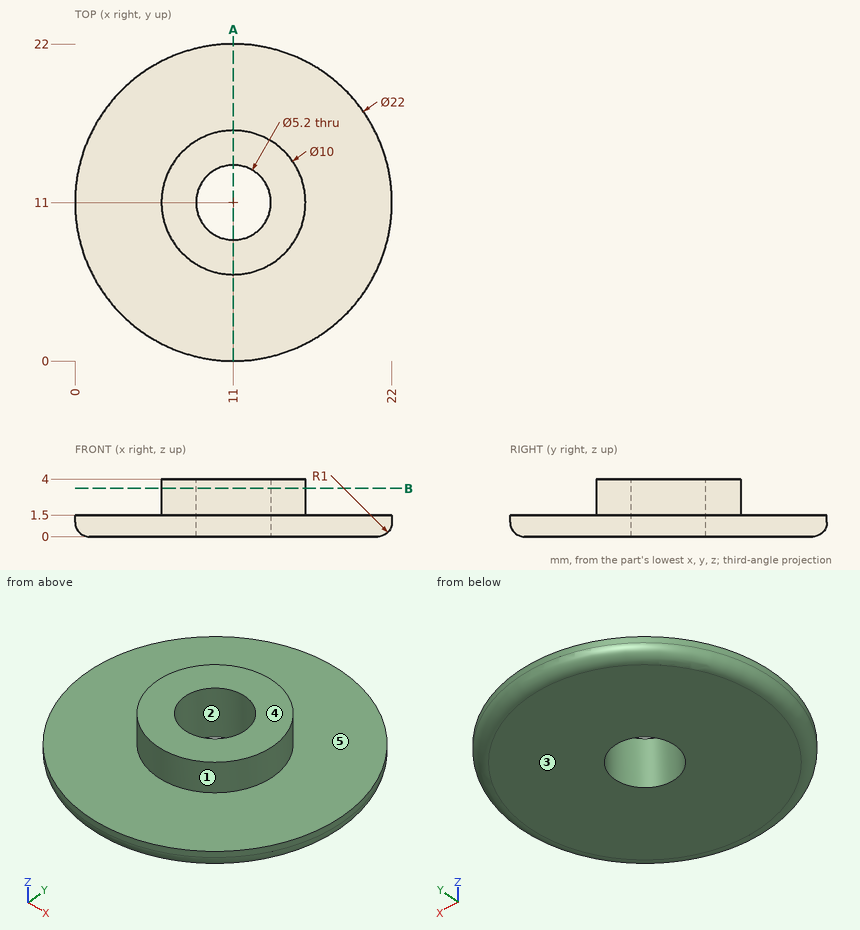
The drawing under review shows one solid part. Ordinate dimensions are in mm from its lowest x, y, z. A direction names the side the tool comes from. Coordinates: 2 decimals unless noted, no trailing zeros. Order: outer loops, then holes, each group sorted by start corner. A loop starts at its lowest first (then second) coordinate and runs counter-clockwise, first axis right, second up. Notation, with made-up numbers: (78, -37) -> (87, -37) arc R20 cw to (87, -26) -> close; hole circle Ø7 at (41, 17.5). An arc over 180 degrees is marked (long way). Return JSON: item names as keys, results as strings.
1. For pin 1 Ø2 at (y, z) = (16.5, 3.5) entering from -X, flat-tipped, find the tip position at first contact; note if it passes through.
Answer block:
{"pin 1": "x = 8.82"}
2. For line 1 (Y direction, x = 11, z = 2.25); line 2 (Y direction, x = 11, z = 0.95); line 3 (Z direction, x = 7.5, y = 6.5), list the stretches that pass through material, from the lowest coordinate up. Write a range as from..to.
Answer block:
{"line 1": "6..8.4, 13.6..16", "line 2": "0..8.4, 13.6..22", "line 3": "0..1.5"}
3. We need section A-A on x = 11. Write out the cut boundary in (y, z).
Answer block:
{"outline": "(0, 1) arc R1 ccw to (1, 0) -> (8.4, 0) -> (8.4, 4) -> (6, 4) -> (6, 1.5) -> (0, 1.5) -> close; (13.6, 0) -> (21, 0) arc R1 ccw to (22, 1) -> (22, 1.5) -> (16, 1.5) -> (16, 4) -> (13.6, 4) -> close"}
4. Machinability: for the marked faces 4 and 5, which of the approach directions +Z, -Z, +X, -X, +Y, -Y give a long, thin tool a straight path to every point of the face, cutting with its end or side? Answer none if there is none.
Answer block:
{"face 4": "+Z, +X, -X, +Y, -Y", "face 5": "+Z"}
5. We need section B-B on z = 3.35. Write out the cut boundary in (x, y).
Answer block:
{"outline": "circle Ø10 at (11, 11); hole circle Ø5.2 at (11, 11)"}
6. The part is to be moulded in two halves that separate along X. For the marked faces 1, 2 and 3, say which applies: +X half, -X half, draft (parallel to the pull), parting line (faces both ways), or undercut.
Answer block:
{"face 1": "parting line", "face 2": "undercut", "face 3": "draft"}
